For this review, use the dimensioned drawing (mm, ordinates from the lowest corner) and the shaded views. A direction names the side the tool comes from. Give positions to 0.01 mm unless a question says otherwise; leave off trailing zeros. Write each loop counter-clockwise with the first axis right and the second up, starting at its lowest first coordinate (ties: lowest second). Pieces come first, ordered by that corner, then holes. Notation, with made-up numbers: M 32,73.5 L 78,73.5 A17 cw 78,79.5 Z; hole C 54,37.5 d1. An arc over 180 degrees is marked long. Answer in a Markdown table with one row per item.
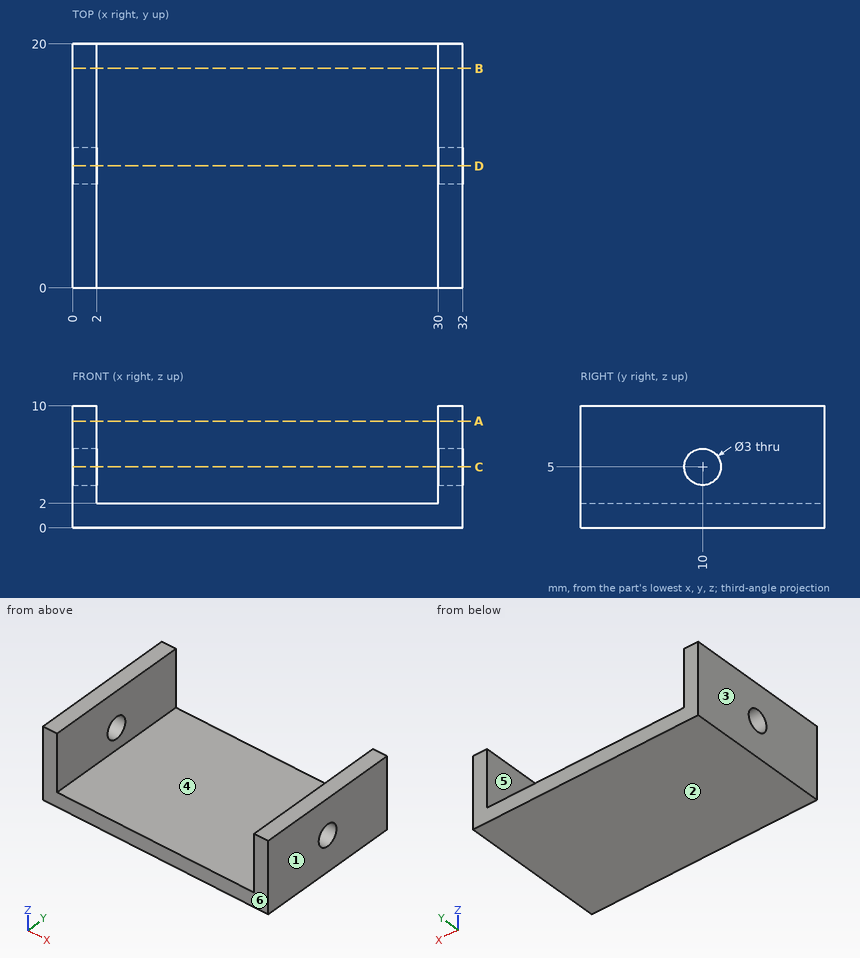
1) Add section A-A (z = 8.75). Write out the cut boundary in (x, y), and give its area (3 significant figures).
Geometry says:
| item | result |
|---|---|
| outline | M 0,0 L 2,0 L 2,20 L 0,20 Z; M 30,0 L 32,0 L 32,20 L 30,20 Z |
| area | 80.0 mm^2 |
2) For the marked faces 5 and 6, list the 3-axis set-ups (+Z, -Z, +X, -X, +Y, -Y) from which the entire face can be reached by the end or side of a thin tool; tool diameter is ignored.
Geometry says:
| item | result |
|---|---|
| face 5 | +Z, +Y, -Y |
| face 6 | +Z, -Z, +X, -X, -Y |
3) Insertion check: P1, Ø1, axis at x = 12.5, y = 3.5, coming from the -Z side; P2, Ø1.8, axis at y = 10, z = 5, coming from the -X side. Each pin has a flat end and moves straight along its axis. Give the tip position at first contact, or say it passes through.
Geometry says:
| item | result |
|---|---|
| P1 | z = 0 |
| P2 | through |
4) Add section D-D (y = 10). Write out the cut boundary in (x, z).
Geometry says:
| item | result |
|---|---|
| outline | M 0,0 L 32,0 L 32,3.5 L 30,3.5 L 30,2 L 2,2 L 2,3.5 L 0,3.5 Z; M 0,6.5 L 2,6.5 L 2,10 L 0,10 Z; M 30,6.5 L 32,6.5 L 32,10 L 30,10 Z |
5) To check wall thickness, follow probe 1 along X at (y, z) = (10, 8); probe 2 along Z at (x, y) = (31, 10); probe 3 along Y at (x, z) = (0.7, 5). State the ranges of each line that lie inside material, in increasing order. Write a range as [from, to].
Geometry says:
| item | result |
|---|---|
| probe 1 | [0, 2], [30, 32] |
| probe 2 | [0, 3.5], [6.5, 10] |
| probe 3 | [0, 8.5], [11.5, 20] |
6) Add section C-C (z = 5). Write out the cut boundary in (x, y), and give its area (3 significant figures).
Geometry says:
| item | result |
|---|---|
| outline | M 0,0 L 2,0 L 2,8.5 L 0,8.5 Z; M 0,11.5 L 2,11.5 L 2,20 L 0,20 Z; M 30,0 L 32,0 L 32,8.5 L 30,8.5 Z; M 30,11.5 L 32,11.5 L 32,20 L 30,20 Z |
| area | 68.0 mm^2 |
7) The part is to be moulded in two halves that separate along X. For the marked faces 1, 2, 3 and 4, say which applies: released by +X, released by -X, zero draft, split by the parting line, or undercut.
Geometry says:
| item | result |
|---|---|
| face 1 | released by +X |
| face 2 | zero draft |
| face 3 | released by -X |
| face 4 | undercut |
8) Add section B-B (y = 18). Write out the cut boundary in (x, z), and give its area (3 significant figures).
Geometry says:
| item | result |
|---|---|
| outline | M 0,0 L 32,0 L 32,10 L 30,10 L 30,2 L 2,2 L 2,10 L 0,10 Z |
| area | 96.0 mm^2 |
